```python
from build123d import *

# Parameters (mm, degrees)
SKETCH1_R           = 28.097988
BOSS_EXTRUDE1_DEPTH = 6.35
SKETCH2_R           = 1.016
SKETCH2_R_2         = 2.9
CUT_EXTRUDE1_DEPTH  = 6.35


with BuildPart() as part:
    # Sketch1 → Boss-Extrude1 (new body)
    with BuildSketch(Plane.XY):
        Circle(SKETCH1_R)
    extrude(amount=BOSS_EXTRUDE1_DEPTH)

    # Sketch2 → Cut-Extrude1 (cut)
    with BuildSketch(Plane(origin=(0, 0, 0), x_dir=(-1, 0, 0), z_dir=(0, 0, -1))):
        with Locations((-13.220714373, -2.876388616)):
            Circle(SKETCH2_R)
        with Locations((-16.152136629, -3.514168797)):
            Circle(SKETCH2_R)
        with Locations((-10.289292117, -2.238608435)):
            Circle(SKETCH2_R)
        with Locations((-7.357869862, -1.600828254)):
            Circle(SKETCH2_R)
        with Locations((7.357869862, 1.600828254)):
            Circle(SKETCH2_R)
        with Locations((10.289292117, 2.238608435)):
            Circle(SKETCH2_R)
        with Locations((13.220714373, 2.876388616)):
            Circle(SKETCH2_R)
        with Locations((16.152136629, 3.514168797)):
            Circle(SKETCH2_R)
        Circle(SKETCH2_R_2)
    extrude(amount=-CUT_EXTRUDE1_DEPTH, mode=Mode.SUBTRACT)


solid = part.part
```
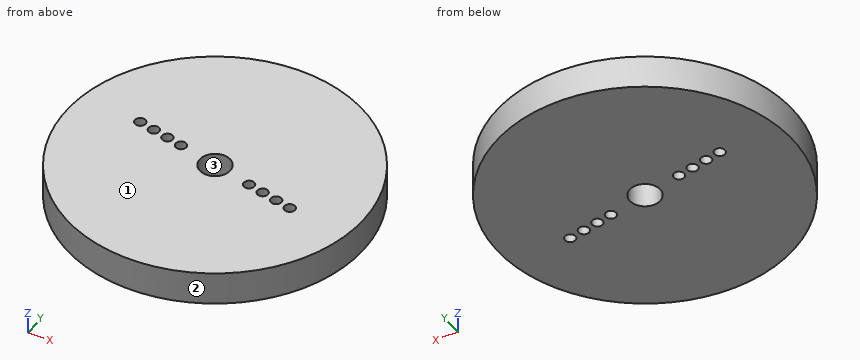
Read the model definition and answer for the solid it produces. Units are mm, in the model's axes. Face numbers are marked on the shaded views. Give positions to 0.01 mm unless a question says otherwise; leave off trailing zeros. Write each loop counter-clockwise with the first axis right and the second up, starting at its lowest first coordinate (ties: lowest second). Pieces come first, ordered by that corner, then holes. Notation, with made-up numbers: M 81,51 L 96,51 A16 cw 96,80 Z; hole C -24,19 d6. An arc over 180 degrees is marked long. Put each result on its own line as item: value. Start each with the question number.
1. For a pull along X with two mould halves and no side action, classify the marked faces 1, 2 and 3 as released by +X, released by -X, zero draft, split by the parting line, or undercut.
2. The part is cut by section B-B, the plane z = 3.25. Give the number of separate pieces and of enclosed holes in the cut face, and give its area (3 significant figures).
3. The part is cut by section A-A, the plane x = 0. Give the vertices of the cut face in (y, z).
4. Each of these flat-tipped pins is pushed along its axis until it touches: pin 1 Ø3 at (y, z) = (-13.5, 3) entering from +X; pin 2 Ø1.8 at (x, y) = (16.15, -3.51) entering from -Z; pin 3 Ø1.5 at (x, z) = (10.5, 1) entering from -Y. Where does it stop, or does it pass through?
5. Consider line 1 along Y through (x, z) = (0, 3); line 2 along X through (y, z) = (-2, 1); line 3 along X through (y, z) = (-16, 1.75). Determine where each line is inside the solid, lowest interval first.
6. The part is cut by section D-D, the plane y = 16. Give the vertices of the cut face in (x, z), and give its area (3 significant figures).
7. The part is cut by section C-C, the plane x = 10.5. Give the vertices of the cut face in (y, z).
Final values:
1. face 1: zero draft
1. face 2: split by the parting line
1. face 3: undercut
2. separate pieces: 1
2. enclosed holes: 9
2. area: 2,430 mm²
3. outline: M -28.1,0 L -2.9,0 L -2.9,6.35 L -28.1,6.35 Z; M 2.9,0 L 28.1,0 L 28.1,6.35 L 2.9,6.35 Z
4. pin 1: stops at x = 25.41
4. pin 2: passes through
4. pin 3: stops at y = -26.35
5. line 1: y = -28.1 to -2.9, 2.9 to 28.1
5. line 2: x = -28.03 to -2.1, 2.1 to 6.42, 8.29 to 9.3, 11.28 to 12.71, 13.73 to 28.03
5. line 3: x = -23.1 to 23.1
6. outline: M -23.1,0 L 23.1,0 L 23.1,6.35 L -23.1,6.35 Z
6. area: 293 mm²
7. outline: M -26.06,0 L -3.23,0 L -3.23,6.35 L -26.06,6.35 Z; M -1.24,0 L 26.06,0 L 26.06,6.35 L -1.24,6.35 Z
